```python
from build123d import *

# Parameters (mm, degrees)
BOSS_EXTRUDE1_DEPTH = 8
BOSS_EXTRUDE2_DEPTH = 5
FILLET1_R           = 8
SKETCH3_R           = 1.625
CUT_EXTRUDE1_DEPTH  = 52.963032648
SKETCH4_R           = 3
CUT_EXTRUDE2_DEPTH  = 1
SKETCH5_W           = 2
SKETCH5_H           = 17.649761518
BOSS_EXTRUDE3_DEPTH = 3
FILLET2_R           = 2
CHAMFER1_SIZE       = 0.2
CHAMFER1_SIZE2      = 0.346410162


with BuildPart() as part:
    # Sketch1 → Boss-Extrude1 (new body)
    with BuildSketch(Plane(origin=(0, 0, 0), x_dir=(1, 0, 0), z_dir=(0, 1, 0))):
        with BuildLine():
            Line((-16, -15.658779245), (-16, -44.520095044))
            Line((-16, -44.520095044), (-11, -44.520095044))
            Line((-11, -44.520095044), (-11, -18.904054542))
            Line((-11, -18.904054542), (0, -14))
            ThreePointArc((0, -14), (9.899494937, 9.899494937), (-14, 0))
            Line((-14, 0), (-9, 0))
            ThreePointArc((-9, 0), (6.691765492, 6.018328223), (-0.951050089, -8.949609138))
            Line((-0.951050089, -8.949609138), (-16, -15.658779245))
        make_face()
    extrude(amount=BOSS_EXTRUDE1_DEPTH)

    # Sketch2 → Boss-Extrude2 (add)
    with BuildSketch(Plane.ZY.offset(16)):
        with BuildLine():
            Line((44.520095044, 0), (44.520095044, -9.649761518))
            Line((44.520095044, -9.649761518), (33.520095044, -9.649761518))
            ThreePointArc((33.520095044, -9.649761518), (27.783236203, -2.635329296), (19.113239186, 0))
            Line((19.113239186, 0), (44.520095044, 0))
        make_face()
    extrude(amount=-BOSS_EXTRUDE2_DEPTH)

    # Fillet1
    fillet1_edges = [part.edges().sort_by_distance(p)[0] for p in [
        (0, 4, 14),
        (-11, 4, 18.904054542),
    ]]
    fillet(fillet1_edges, radius=FILLET1_R)
    fillet1_2_edges = [part.edges().sort_by_distance(p)[0] for p in [
        (-0.951050089, 4, 8.949609138),
        (-16, 4, 15.658779245),
    ]]
    fillet(fillet1_2_edges, radius=FILLET1_R)

    # Sketch3 → Cut-Extrude1 (cut, through all)
    with BuildSketch(Plane(origin=(-11, 0, 0), x_dir=(0, 0, -1), z_dir=(1, 0, 0))):
        with Locations((-40.320095044, 4)):
            Circle(SKETCH3_R)
        with Locations((-40.320095044, -6)):
            Circle(SKETCH3_R)
    extrude(amount=-CUT_EXTRUDE1_DEPTH, mode=Mode.SUBTRACT)

    # Sketch4 → Cut-Extrude2 (cut)
    with BuildSketch(Plane(origin=(-11, 0, 0), x_dir=(0, 0, -1), z_dir=(1, 0, 0))):
        with Locations((-40.320095044, 4)):
            Circle(SKETCH4_R)
        with Locations((-40.320095044, -6)):
            Circle(SKETCH4_R)
    extrude(amount=-CUT_EXTRUDE2_DEPTH, mode=Mode.SUBTRACT)

    # Sketch5 → Boss-Extrude3 (add)
    with BuildSketch(Plane.ZY.offset(16)):
        with Locations((35.520095044, -0.824880759)):
            Rectangle(SKETCH5_W, SKETCH5_H)
    extrude(amount=BOSS_EXTRUDE3_DEPTH)

    # Fillet2
    fillet2_edges = [part.edges().sort_by_distance(p)[0] for p in [
        (-16, -0.824880759, 34.520095044),
    ]]
    fillet(fillet2_edges, radius=FILLET2_R)

    # Chamfer1
    chamfer1_edges = [part.edges().sort_by_distance(p)[0] for p in [
        (-16.585786438, 8, 33.934308606),
        (-11.5, 8, 0),
        (6.237696494, 8, -6.48776868),
        (-13.5, 8, 44.520095044),
        (-6.923574229, 8, 11.612298605),
        (-11, 8, 34.308295031),
        (-3.815638997, 8, 15.70110016),
        (9.46618809, 8, -10.314615022),
        (-16, 8, 26.685657382),
        (-14.710444905, 8, 16.495771504),
        (-1.150763069, 8, 9.19633523),
        (-0.11525428, 8, 14.172981147),
        (-9.710444905, 8, 19.741046801),
        (-16, 8, 40.520095044),
        (-17.5, 8, 36.520095044),
        (-18.5, 8, 34.520095044),
        (-19, 8, 35.520095044),
    ]]
    chamfer1_side = [part.faces().sort_by_distance(p)[0] for p in [
        (-15.328166574, 8, 26.685657382),
    ]]
    chamfer(chamfer1_edges, length=CHAMFER1_SIZE, length2=CHAMFER1_SIZE2, reference=chamfer1_side[0])


solid = part.part
```
The model under review builds one solid part; all positions refer to its coordinate system, in mm. A direction names the side the tool comes from. Coordinates: 2 decimals unless noted, no trailing zeros. Write each loop counter-clockwise with the first axis right and the second up, starting at its lowest first coordinate (ties: lowest second). Pieces come first, ordered by that corner, then holes.
1) Clearance check with flat-ended pins moving along their axes: pin 1 Ø9 at (y, z) = (-3.5, 41.5) entering from -X; pin 2 Ø5 at (x, z) = (-10, 22.5) entering from -Y; pin 3 Ø1.9 at (y, z) = (-6, 40.32) entering from +X; pin 4 Ø8 at (x, y) = (4.5, 0) entering from -Z. State where each tip first meets the part, or that it passes through.
2) The part is to be moulded in two halves that separate along Y. For faces 1 (the face through (-13.97, 4.49, 38.77)), 2 (the face through (-6.9, 3.8, 11.6)), 3 (the face through (-9.81, 7.79, 19.75)), 4 (the face through (-11.493, -5.868, 43.317)), say which applies: pulls with the +Y half, pulls with the -Y half, needs draft (parallel to the pull), parting line crosses it, or undercut.
3) We need section A-A on y = -5. State the section outline as (x, z) points.
4) To check wall thickness, follow probe 1 along X at (y, z) = (3.25, 36); probe 2 along Z at (x, y) = (-15, 2.75); probe 3 along Y at (x, z) = (-7.5, 12.5). State the ranges of each line that lie inside material, in increasing order.
5) We need section C-C on x = -15. Count the separate pieces of the cut face and the enclosed holes in it, then the cut area to 3 significant figures.
6) Machinability: for faces 5 (the face through (-14.574, 7.863, 16.508)), 6 (the face through (-17, -1, 36.52)), 7 (the face through (3, 0, 9)), 8 (the face through (-16, 2, 28)), which of the approach directions +Z, -Z, +X, -X, +Y, -Y give a long, thin tool a straight path to every point of the face, cutting with its end or side? Answer none if there is none.
7) We need section B-B on y = 4. State the section outline as (x, z) points, then the cut area to 3 significant figures.
Answer list:
1. pin 1: stops at x = -16
1. pin 2: stops at y = -1.07
1. pin 3: passes through
1. pin 4: stops at z = -13.99
2. face 1: undercut
2. face 2: needs draft
2. face 3: pulls with the +Y half
2. face 4: undercut
3. outline: (-19, 34.52) - (-18, 34.52) arc R2 cw to (-16, 32.52) - (-16, 30.55) - (-11, 30.55) - (-11, 37.49) - (-12, 37.49) - (-12, 39.04) - (-16, 39.04) - (-16, 36.52) - (-19, 36.52) - close; (-16, 41.6) - (-12, 41.6) - (-12, 43.15) - (-11, 43.15) - (-11, 44.52) - (-16, 44.52) - close
4. probe 1: x = -19 to -11
4. probe 2: z = 16.98 to 39.28, 41.36 to 44.52
4. probe 3: y = 0 to 8
5. separate pieces: 1
5. enclosed holes: 2
5. area: 348 mm2
6. face 5: -X, +Y
6. face 6: +Z, -X, +Y, -Y
6. face 7: -Z, +X, -X, -Y
6. face 8: -Z, -X, +Y, -Y
7. outline: (-19, 34.52) - (-18, 34.52) arc R2 cw to (-16, 32.52) - (-16, 20.85) arc R8 ccw to (-11.26, 13.54) - (-2.59, 9.68) arc R8 ccw to (0.35, 8.99) arc R9 cw (long way) to (-9, 0) - (-14, 0) arc R14 ccw (long way) to (1.2, 13.95) arc R8 cw to (-1.37, 14.61) - (-6.26, 16.79) arc R8 cw to (-11, 24.1) - (-11, 37.32) - (-12, 37.32) - (-12, 38.7) - (-16, 38.7) - (-16, 36.52) - (-19, 36.52) - close; (-16, 41.95) - (-12, 41.95) - (-12, 43.32) - (-11, 43.32) - (-11, 44.52) - (-16, 44.52) - close
7. area: 469 mm2
